The model under review builds one solid part; all positions refer to its coordinate system, in mm. Face numbers are marked on the shaded views. Coordinates: 2 decimals unless noted, no trailing zeros. Order: outer loops, then holes, each group sorted by start corner. A loop starts at its lowest first (then second) coordinate and runs counter-clockwise, first axis right, second up.
```python
from build123d import *

# Parameters (mm, degrees)
F0_W     = 100
F0_H     = 200
F1_DEPTH = 13
F3_W     = 88.300774
F3_H     = 187.619995
F4_DEPTH = 10
F5_R     = 5
F6_R     = 5
F7_R     = 5
F8_R     = 5
F9_R     = 5
F10_R    = 5
F11_R    = 5
F12_R    = 5
F13_R    = 5


with BuildPart() as f1:
    # F0 (on Top) → F1 (new body)
    with BuildSketch(Plane.XY):
        with Locations((50, 100)):
            Rectangle(F0_W, F0_H)
    extrude(amount=F1_DEPTH)

    # F3 (on face) → F4 (cut)
    with BuildSketch(Plane.XY.offset(13)):
        with Locations((49.800339, 99.72308)):
            Rectangle(F3_W, F3_H)
    extrude(amount=-F4_DEPTH, mode=Mode.SUBTRACT)

    # F5
    f5_edges = [f1.edges().sort_by_distance(p)[0] for p in [
        (100, 200, 6.5),
    ]]
    fillet(f5_edges, radius=F5_R)

    # F6
    f6_edges = [f1.edges().sort_by_distance(p)[0] for p in [
        (0, 200, 6.5),
    ]]
    fillet(f6_edges, radius=F6_R)

    # F7
    f7_edges = [f1.edges().sort_by_distance(p)[0] for p in [
        (100, 0, 6.5),
    ]]
    fillet(f7_edges, radius=F7_R)

    # F8
    f8_edges = [f1.edges().sort_by_distance(p)[0] for p in [
        (0, 0, 6.5),
    ]]
    fillet(f8_edges, radius=F8_R)

    # F9
    f9_edges = [f1.edges().sort_by_distance(p)[0] for p in [
        (5.649952, 5.913083, 8),
    ]]
    fillet(f9_edges, radius=F9_R)

    # F10
    f10_edges = [f1.edges().sort_by_distance(p)[0] for p in [
        (5.649952, 193.533078, 8),
    ]]
    fillet(f10_edges, radius=F10_R)

    # F11
    f11_edges = [f1.edges().sort_by_distance(p)[0] for p in [
        (93.950726, 193.533078, 8),
    ]]
    fillet(f11_edges, radius=F11_R)

    # F12
    f12_edges = [f1.edges().sort_by_distance(p)[0] for p in [
        (93.950726, 5.913083, 8),
    ]]
    fillet(f12_edges, radius=F12_R)

    # F13
    f13_edges = [f1.edges().sort_by_distance(p)[0] for p in [
        (0, 100, 0),
    ]]
    fillet(f13_edges, radius=F13_R)


solid = f1.part
```
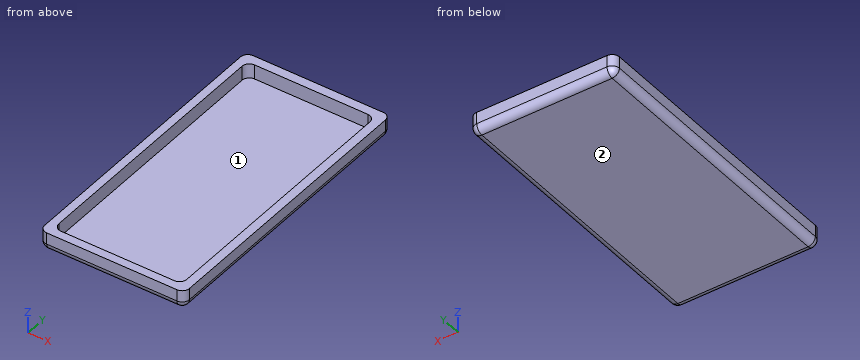
(1) Wall thickness on probe 1 along Y at (x, z) = (19.5, 6); probe 2 along X at (y, z) = (189, 5); probe 3 along X at (y, z) = (86.5, 12): over which ranges is each line inside the solid? List them lowest first.
A:
probe 1: y = 0 to 5.91, 193.53 to 200
probe 2: x = 0 to 5.67, 93.93 to 100
probe 3: x = 0 to 5.65, 93.95 to 100
(2) For pin 1 Ø12 at (x, y) = (80, 177) entering from +Z; pin 2 Ø6 at (y, z) = (63, 1.5) entering from -X, all flat-tipped, find the tip position at first contact; note any pin that passes through.
A:
pin 1: stops at z = 3
pin 2: stops at x = 0.03
(3) Draft analysis for pull direction X (two halves, no side actions). For the marked faces 1 and 2, state which applies: released by +X, released by -X, zero draft, split by the parting line, or undercut.
A:
face 1: undercut
face 2: zero draft
(4) We need section B-B, the plane x = 35. Write out the cut boundary in (y, z).
A:
outline: (0, 5) arc R5 ccw to (5, 0) - (195, 0) arc R5 ccw to (200, 5) - (200, 13) - (193.53, 13) - (193.53, 3) - (5.91, 3) - (5.91, 13) - (0, 13) - close
(5) We need section C-C, the plane y = 136. Write out the cut boundary in (x, z), and give its area (3 significant figures).
A:
outline: (0, 5) arc R5 ccw to (5, 0) - (95, 0) arc R5 ccw to (100, 5) - (100, 13) - (93.95, 13) - (93.95, 3) - (5.65, 3) - (5.65, 13) - (0, 13) - close
area: 406 mm2
(6) We need section A-A, the plane z = 9.25. Write out the cut boundary in (x, y).
A:
outline: (0, 5) arc R5 ccw to (5, 0) - (95, 0) arc R5 ccw to (100, 5) - (100, 195) arc R5 ccw to (95, 200) - (5, 200) arc R5 ccw to (0, 195) - close; hole (5.65, 10.91) arc R5 ccw to (10.65, 5.91) - (88.95, 5.91) arc R5 ccw to (93.95, 10.91) - (93.95, 188.53) arc R5 ccw to (88.95, 193.53) - (10.65, 193.53) arc R5 ccw to (5.65, 188.53) - close
